from build123d import *

# Parameters (mm, degrees)
F0_R     = 1.75
F1_DEPTH = 2.5


with BuildPart() as f1:
    # F0 (on Top) → F1 (new body)
    with BuildSketch(Plane.XY):
        Polygon((-27.05, 8), (-20.55, 0), (-20.55, -60), (0, -60), (20.55, -60), (20.55, 0), (27.05, 8), (27.05, 20.4), (0, 20.4), (-27.05, 20.4), align=None)
        with Locations((-21.8, 5.5)):
            Circle(F0_R, mode=Mode.SUBTRACT)
        with Locations((21.8, 5.5)):
            Circle(F0_R, mode=Mode.SUBTRACT)
    extrude(amount=F1_DEPTH)


solid = f1.part
The model under review builds one solid part; all positions refer to its coordinate system, in mm. A direction names the side the tool comes from. Give positions to 0.01 mm unless a question says otherwise; leave off trailing zeros. Write each loop counter-clockwise with the first axis right and the second up, starting at its lowest first coordinate (ties: lowest second). Pieces come first, ordered by that corner, then holes.
1. Wall thickness on L1, parallel to X at y = -15.5, z = 1.9; L2, parallel to Y at x = -22, z = 0.25; L3, parallel to Y at x = -21.8, z = 0.9: over which ranges is each line inside the solid? List them lowest first.
2. Tool access review of faces 4 (the cylindrical face through (-20.183, 4.83, 1.232)), 5 (the flat face through (-20.55, -30, 1)), 6 (the flat face through (20.55, -30, 1)): name each direction out of +Z, -Z, +X, -X, +Y, -Y from which nothing blocks a thin tool from reaching the whole face with its end or side.
3. Add section A-A, the plane z = 1.5. Write out the cut boundary in (x, y), plus the area to 3 significant figures.
4. Add section B-B, the plane x = -21.8. Write out the cut boundary in (y, z).
5. Draft analysis for pull direction Y (two halves, no side actions). For faces 1 (the cylindrical face through (23.417, 4.83, 1.232)), 2 (the flat face through (0, -19, 0)), 3 (the flat face through (0, -60, 1)), state which applies: +Y half, -Y half, draft (parallel to the pull), parting line (faces both ways), or undercut.
6. For P1, Ø1.2, axis at y = -35.5, z = 1, coming from the -X side, flat-tipped, find the tip position at first contact; note if it passes through.
7. Add section C-C, the plane y = -46.5. Write out the cut boundary in (x, z).
Worked answers:
1. L1: x = -20.55 to 20.55
1. L2: y = 1.78 to 3.76, 7.24 to 20.4
1. L3: y = 1.54 to 3.75, 7.25 to 20.4
2. face 4: +Z, -Z
2. face 5: +Z, -Z, -X, -Y
2. face 6: +Z, -Z, +X, -Y
3. outline: (-27.05, 8) - (-20.55, 0) - (-20.55, -60) - (20.55, -60) - (20.55, 0) - (27.05, 8) - (27.05, 20.4) - (-27.05, 20.4) - close; hole circle Ø3.5 at (-21.8, 5.5); hole circle Ø3.5 at (21.8, 5.5)
3. area: 3,500 mm2
4. outline: (1.54, 0) - (3.75, 0) - (3.75, 2.5) - (1.54, 2.5) - close; (7.25, 0) - (20.4, 0) - (20.4, 2.5) - (7.25, 2.5) - close
5. face 1: undercut
5. face 2: draft
5. face 3: -Y half
6. P1: stops at x = -20.55
7. outline: (-20.55, 0) - (20.55, 0) - (20.55, 2.5) - (-20.55, 2.5) - close
